```python
from build123d import *

# Parameters (mm, degrees)
SKETCH1_W                       = 120
SKETCH1_H                       = 60
BOSS_EXTRUDE1_DEPTH             = 22.5
SHELL1_T                        = -1
BOSS_EXTRUDE2_DEPTH             = 45
CUT_EXTRUDE1_DEPTH              = 125.323167592
BOSS_EXTRUDE3_REACH             = 96.877
SKETCH8_R                       = 7.5
BOSS_EXTRUDE3_DIRECTION_2_DEPTH = 18


with BuildPart() as part:
    # Sketch1 → Boss-Extrude1 (new body)
    with BuildSketch(Plane(origin=(0, 0, 0), x_dir=(1, 0, 0), z_dir=(0, 1, 0))):
        Rectangle(SKETCH1_W, SKETCH1_H)
    extrude(amount=BOSS_EXTRUDE1_DEPTH)

    # Shell1
    shell1_openings = [part.faces().sort_by_distance(p)[0] for p in [
        (0, 0, 0),
    ]]
    offset(amount=SHELL1_T, openings=shell1_openings, kind=Kind.INTERSECTION)

    # Sketch2 → Boss-Extrude2 (add)
    with BuildSketch(Plane(origin=(0, 22.5, 0), x_dir=(1, 0, 0), z_dir=(0, 1, 0))):
        with BuildLine():
            Line((-40, 30), (40, 30))
            Line((40, 30), (40, 18))
            Line((40, 18), (20.787496232, 18))
            ThreePointArc((20.787496232, 18), (0, 5.997500139), (-20.787496232, 18))
            Line((-20.787496232, 18), (-40, 18))
            Line((-40, 18), (-40, 30))
        make_face()
    extrude(amount=BOSS_EXTRUDE2_DEPTH)

    # Sketch3 → Cut-Extrude1 (cut, through all)
    with BuildSketch(Plane(origin=(40, 0, 0), x_dir=(0, 0, -1), z_dir=(1, 0, 0))):
        Polygon((24, 67.5), (5.997500139, 67.5), (5.997500139, 37.5), align=None)
    extrude(amount=-CUT_EXTRUDE1_DEPTH, mode=Mode.SUBTRACT)

    # Sketch8 → Boss-Extrude3 (add, up to next)
    with BuildSketch(Plane(origin=(0, 7.282369087, 12.135596405), x_dir=(1, 0, 0), z_dir=(0, 0.514548292074691, 0.8574614015353803)), mode=Mode.PRIVATE) as boss_extrude3_sk1:
        with Locations(Location((0, 64.397447073, 0), (0, 0, 51.021392107))):
            Circle(SKETCH8_R)
    boss_extrude3_tool1 = extrude(boss_extrude3_sk1.sketch, amount=-BOSS_EXTRUDE3_REACH, mode=Mode.PRIVATE) - part.part
    add(boss_extrude3_tool1.solids().sort_by_distance((0, 62.500694, -21))[0])

    # Sketch8 → Boss-Extrude3 direction 2 (add)
    with BuildSketch(Plane(origin=(0, 7.282369087, 12.135596405), x_dir=(1, 0, 0), z_dir=(0, 0.514548292074691, 0.8574614015353803))):
        with Locations(Location((0, 64.397447073, 0), (0, 0, 51.021392107))):
            Circle(SKETCH8_R)
    extrude(amount=BOSS_EXTRUDE3_DIRECTION_2_DEPTH)


solid = part.part
```
CAD build for the part. Positions are in the model's coordinates, mm. A direction names the side the tool comes from. Round coordinates to 2 decimals unless told otherwise and drop trailing zeros. Loops run counter-clockwise (first coordinate to the right, second up) from the corner with the lowest first, then second, coordinate; pieces in that order, holes last. Notation, with made-up numbers: M 61,-26.75 L 101,-26.75 A5 cw 101,-18.75 Z; hole C 7.5,-30 d9. An arc over 180 degrees is marked long. Return JSON: item names as keys, results as strings. Group by question number.
(1) Saw through at A-A, the plane z = 5. List the corners of the cut face in (x, y), and give its area (3 significant figures).
(2) Drop flat-ended pins along their axis: P1, Ø21, axis at x = -30.5, y = 40, coming from the +Z side; P2, Ø12, axis at x = 23, z = -6.5, coming from the -Y side; P3, Ø12, axis at y = 38, z = -20, coming from the -X side. Give the stop position or say it passes through.
(3) Saw through at D-D, the plane y = 28.5. List the corners of the cut face in (x, z) (1 decimal), and give its area (3 significant figures).
(4) Saw through at B-B, the plane x = -42.5. List the corners of the cut face in (y, z), and give its area (3 significant figures).
(5) Mould opens along X. For faces 1 (the flat face through (-40, 45, -24)), 2 (the flat face through (40, 45, -24)), 3 (the flat face through (1, 67.5, -28)), 4 (the flat face through (-1, 11, -29)) say: +X half, -X half, draft (parallel to the pull), parting line (faces both ways), or undercut.
(6) Tool access for faces 5 (the cylindrical face through (0.4, 32, -6)), 6 (the flat face through (-30, 40, -18)), 7 (the flat face through (31, 40, -18)), 8 (the flat face through (-59, 11, 0)): list every direction of +Z, -Z, +X, -X, +Y, -Y with a clear straight run to the whole face (end or side of a thin tool).
(7) Wall check: probe 1 along Z at (x, y) = (45, 11.5); probe 2 along X at (y, z) = (16.5, -26); probe 3 along Z at (x, y) = (-33.5, 56). Give the ranges that are in metal, low to high. Write a range as [from, to].
(8) Saw through at C-C, the plane y = 11. List the corners of the cut face in (x, z), and give its area (3 significant figures).
Answer list:
{
 "1": {"outline": "M -60,0 L -59,0 L -59,21.5 L 59,21.5 L 59,0 L 60,0 L 60,22.5 L -60,22.5 Z", "area": "163 mm2"},
 "2": {"P1": "z = -16.73", "P2": "y = 21.5", "P3": "x = -40"},
 "3": {"outline": "M -40,-30 L 40,-30 L 40,-18 L 20.8,-18 A24 ccw -20.8,-18 L -40,-18 Z", "area": "1,310 mm2"},
 "4": {"outline": "M 0,-30 L 22.5,-30 L 22.5,30 L 0,30 L 0,29 L 21.5,29 L 21.5,-29 L 0,-29 Z", "area": "103 mm2"},
 "5": {"face 1": "-X half", "face 2": "+X half", "face 3": "draft", "face 4": "undercut"},
 "6": {"face 5": "+Z", "face 6": "+Z, -X, +Y", "face 7": "+Z, +X, +Y", "face 8": "-Y"},
 "7": {"probe 1": "[-30, -29], [29, 30]", "probe 2": "[-60, -59], [59, 60]", "probe 3": "[-30, -18]"},
 "8": {"outline": "M -60,-30 L 60,-30 L 60,30 L -60,30 Z; hole M -59,-29 L 59,-29 L 59,29 L -59,29 Z", "area": "356 mm2"}
}
